from build123d import *

# Parameters (mm, degrees)
SKETCH_1_W          = 170
SKETCH_1_H          = 80
EXTRUDE_1_DEPTH     = 5
SKETCH_2_R          = 7.75
SKETCH_2_R_2        = 3.25
SKETCH_2_W          = 79.5
SKETCH_2_H          = 51.5
CUT_EXTRUDE_1_DEPTH = 151.961816214
SKETCH_5_W          = 170
SKETCH_5_H          = 25
EXTRUDE_3_DEPTH     = 5
SKETCH_7_R          = 2.75
CUT_EXTRUDE_4_DEPTH = 165.330739172
SKETCH_9_R          = 1
CUT_EXTRUDE_5_DEPTH = 153.19878434
SKETCH_10_R         = 1.75
CUT_EXTRUDE_6_DEPTH = 153.936163005


with BuildPart() as part:
    # 草图1 → 凸台-拉伸1 (new body)
    with BuildSketch(Plane(origin=(0, 0, 0), x_dir=(1, 0, 0), z_dir=(0, 1, 0))):
        with Locations((57.142857143, -10.595238095)):
            Rectangle(SKETCH_1_W, SKETCH_1_H)
    extrude(amount=EXTRUDE_1_DEPTH)

    # 草图2 → 切除-拉伸1 (cut, through all)
    with BuildSketch(Plane(origin=(0, 5, 0), x_dir=(1, 0, 0), z_dir=(0, 1, 0))):
        with Locations(Location((-12.857142857, 9.404761905, 0), (0, 0, 270))):
            Circle(SKETCH_2_R)
        with Locations(Location((-12.857142857, -25.595238095, 0), (0, 0, 270))):
            Circle(SKETCH_2_R)
        with Locations(Location((127.142857143, -6.659623692, 0), (0, 0, 270))):
            Circle(SKETCH_2_R_2)
        with Locations(Location((127.142857143, -30.595238095, 0), (0, 0, 270))):
            Circle(SKETCH_2_R)
        with Locations((57.142857143, -10.595238095)):
            Rectangle(SKETCH_2_W, SKETCH_2_H)
    extrude(amount=-CUT_EXTRUDE_1_DEPTH, mode=Mode.SUBTRACT)

    # 草图5 → 凸台-拉伸3 (add)
    with BuildSketch(Plane(origin=(0, 0, 50.595238095), x_dir=(-1, 0, 0), z_dir=(0, 0, -1))):
        with Locations((-57.142857143, -7.5)):
            Rectangle(SKETCH_5_W, SKETCH_5_H)
    extrude(amount=EXTRUDE_3_DEPTH)

    # 草图7 → 切除-拉伸4 (cut, through all)
    with BuildSketch(Plane.XY.offset(50.595238095)):
        with Locations((-2.857142857, -7.5)):
            Circle(SKETCH_7_R)
        with Locations((117.142857143, -7.5)):
            Circle(SKETCH_7_R)
    extrude(amount=-CUT_EXTRUDE_4_DEPTH, mode=Mode.SUBTRACT)

    # 草图9 → 切除-拉伸5 (cut, through all)
    with BuildSketch(Plane.XZ):
        with Locations(Location((14.142857143, -18.904761905, 0), (0, 0, 270))):
            Circle(SKETCH_9_R)
        with Locations(Location((100.142857143, -18.904761905, 0), (0, 0, 270))):
            Circle(SKETCH_9_R)
        with Locations(Location((100.142857143, 40.095238095, 0), (0, 0, 270))):
            Circle(SKETCH_9_R)
        with Locations(Location((14.142857143, 40.095238095, 0), (0, 0, 270))):
            Circle(SKETCH_9_R)
    extrude(amount=-CUT_EXTRUDE_5_DEPTH, mode=Mode.SUBTRACT)

    # 草图10 → 切除-拉伸6 (cut, through all)
    with BuildSketch(Plane(origin=(0, 5, 0), x_dir=(1, 0, 0), z_dir=(0, 1, 0))):
        with Locations(Location((-20.857142857, 25.904761905, 0), (0, 0, 270))):
            Circle(SKETCH_10_R)
        with Locations(Location((-20.857142857, -43.191421848, 0), (0, 0, 270))):
            Circle(SKETCH_10_R)
        with Locations(Location((135.142857143, -43.191421848, 0), (0, 0, 270))):
            Circle(SKETCH_10_R)
        with Locations(Location((135.142857143, 25.904761905, 0), (0, 0, 270))):
            Circle(SKETCH_10_R)
    extrude(amount=-CUT_EXTRUDE_6_DEPTH, mode=Mode.SUBTRACT)


solid = part.part
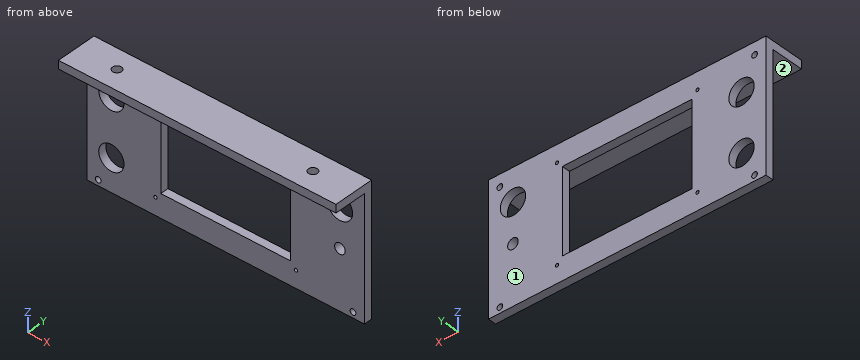
Input: part model. Units: mm. Frame: model coordinates. Face numbers are marked on the shaded views. A direction names the side the tool comes from. Give positions to 0.01 mm unless a question says otherwise; leave off trailing zeros. Order: outer loops, then holes, each group sorted by start corner. A loop starts at its lowest first (then second) coordinate and runs counter-clockwise, first axis right, second up.
Q1. Section A-A on y = -7.5. Output: boundary loops of the cut face in (x, z).
Checked values:
outline: (-27.86, 45.6) - (-5.61, 45.6) - (-5.61, 50.6) - (-27.86, 50.6) - close; (-0.11, 45.6) - (114.39, 45.6) - (114.39, 50.6) - (-0.11, 50.6) - close; (119.89, 45.6) - (142.14, 45.6) - (142.14, 50.6) - (119.89, 50.6) - close
Q2. Contact query for flat-ended pins moving along their axis: pin 1 Ø7 at (x, y) = (117.14, -7.5) entering from -Z; pin 2 Ø4 at (x, z) = (-20.86, -25.9) entering from +Y; pin 3 Ø2 at (x, z) = (124.5, 6.5) entering from -Y. Output: stop coordinate, or through.
Checked values:
pin 1: stops at z = 45.6
pin 2: stops at y = 5
pin 3: stops at y = 0
Q3. Set-up query: the marked faces 1 and 2. Return all of +Z, -Z, +X, -X, +Y, -Y with unobstructed straight access to the full face (end or side cutting, diameter ignored); none if empty.
Checked values:
face 1: +Z, -Z, +X, -X, +Y
face 2: -Z, +X, -X, -Y
Q4. Ray query, probe 1 along Z at (x, y) = (-8, 1); probe 2 along X at (y, z) = (2.25, 27); probe 3 along X at (y, z) = (2.25, -7.5). Return the intervals inside material, ascending.
Checked values:
probe 1: z = -29.4 to -15.44, -3.37 to 19.56, 31.63 to 50.6
probe 2: x = -27.86 to -20.48, -5.24 to 17.39, 96.89 to 120.28, 134.01 to 142.14
probe 3: x = -27.86 to -20.37, -5.34 to 17.39, 96.89 to 142.14
Q5. Section C-C on x = 105. Output: boundary loops of the cut face in (y, z), and give its area (3 significant figures).
Checked values:
outline: (-20, 45.6) - (0, 45.6) - (0, -29.4) - (5, -29.4) - (5, 50.6) - (-20, 50.6) - close
area: 500 mm2
Q6. Section B-B on z = 21. Output: boundary loops of the cut face in (x, y), and give its area (3 significant figures).
Checked values:
outline: (-27.86, 0) - (-19.1, 0) - (-19.1, 5) - (-27.86, 5) - close; (-6.62, 0) - (17.39, 0) - (17.39, 5) - (-6.62, 5) - close; (96.89, 0) - (142.14, 0) - (142.14, 5) - (96.89, 5) - close
area: 390 mm2
